Here's how the part is built. I have some questions about the finished solid (model axes, mm). A direction names the side the tool comes from. Round coordinates to 2 decimals unless told otherwise and drop trailing zeros. Loops run counter-clockwise (first coordinate to the right, second up) from the corner with the lowest first, then second, coordinate; pieces in that order, holes last. Notation, with made-up numbers: M 20.25,-14.5 L 43.25,-14.5 A20 ccw 43.25,-4.5 Z; hole C 59,40.5 d11. An arc over 180 degrees is marked long. Use a Markdown table: item, result.
from build123d import *

# Parameters (mm, degrees)
F0_W     = 44
F0_H     = 44
F0_W_2   = 39
F0_H_2   = 39
F1_DEPTH = 1200
F3_D     = 8.8


# Not quite as in the source:
# - a feature names something its author has since deleted; it is built from what else it names


with BuildPart() as f1:
    # F0 (on Top) → F1 (new body)
    with BuildSketch(Plane.XY):
        Rectangle(F0_W, F0_H)
        Rectangle(F0_W_2, F0_H_2, mode=Mode.SUBTRACT)
    extrude(amount=F1_DEPTH)

    # F3 (through all)
    with Locations(Plane(origin=(-22, 0, 0), x_dir=(0, -1, 0), z_dir=(-1, 0, 0))):
        with Locations((0, 150), (0, 100), (0, 50), (0, 1050), (0, 1150), (0, 1100)):
            Hole(F3_D / 2)


solid = f1.part
1. We'd pull the mould along X, two halves only. Please class faces 1 (the face through (0, 19.5, 592)), 2 (the face through (0, -22, 592)), 3 (the face through (-19.5, 0, 592)), 4 (the face through (-22, 0, 592)): +X half, -X half, draft (parallel to the pull), parting line (faces both ways), or undercut.
Answer sheet:
| item | result |
|---|---|
| face 1 | undercut |
| face 2 | draft |
| face 3 | undercut |
| face 4 | -X half |
2. Which directions (+Z, -Z, +X, -X, +Y, -Y) give clear straight access to the entire face, cutting with the end or side of a thin tool? Please do faces 5 (the face through (0, -19.5, 592)), 6 (the face through (-20, 3, 0)).
Answer sheet:
| item | result |
|---|---|
| face 5 | +Z, -Z |
| face 6 | -Z, +X, -X, +Y, -Y |
3. I need wall thicknesses on probe 1 along Y at (x, z) = (-20, 1050); probe 2 along Y at (x, z) = (2.5, 163). Which ranges of each line are inside material? Lowest first, please. Write a range as from..to.
Answer sheet:
| item | result |
|---|---|
| probe 1 | -22..-4.4, 4.4..22 |
| probe 2 | -22..-19.5, 19.5..22 |
4. For pin 1 Ø7 at (y, z) = (0, 150) entering from +X, with a flat end and sliding along its axis, tell me the tip position at first contact or that it passes through.
Answer sheet:
| item | result |
|---|---|
| pin 1 | through |
5. Imagine slicing it at B-B, the plane y = -12. Write out the boundary of the cut face in (x, z), then the cut area to 3 significant figures.
Answer sheet:
| item | result |
|---|---|
| outline | M -22,0 L -19.5,0 L -19.5,1200 L -22,1200 Z; M 19.5,0 L 22,0 L 22,1200 L 19.5,1200 Z |
| area | 6,000 mm2 |
6. Imagine slicing it at A-A, the plane z = 209. Write out the boundary of the cut face in (x, y), then the cut area to 3 significant figures.
Answer sheet:
| item | result |
|---|---|
| outline | M -22,-22 L 22,-22 L 22,22 L -22,22 Z; hole M -19.5,-19.5 L 19.5,-19.5 L 19.5,19.5 L -19.5,19.5 Z |
| area | 415 mm2 |
